from build123d import *

# Parameters (mm, degrees)
EXTRUDE_1_DEPTH     = 5
SKETCH_3_W          = 100
SKETCH_3_H          = 5
SKETCH_3_W_2        = 5
SKETCH_3_H_2        = 60
EXTRUDE_2_DEPTH     = 55
SKETCH_4_W          = 60
SKETCH_4_H          = 5
EXTRUDE_3_DEPTH     = 100
CUT_EXTRUDE_1_REACH = 89.07
FILLET_2_R          = 10
FILLET_3_R          = 10
FILLET_4_R          = 5
FILLET_5_R          = 2
CUT_EXTRUDE_2_REACH = 85.703
SKETCH_6_R          = 1.65
CUT_EXTRUDE_START   = -50
CUT_EXTRUDE_3_DEPTH = 50
EXTRUDE_4_DEPTH     = 60
SKETCH_10_W         = 7.5
SKETCH_10_H         = 18
CUT_EXTRUDE_4_DEPTH = 5


# Read off the part's stored shape, not the designer's step: 切除-拉伸3
with BuildPart() as part:
    # 草图1 → 凸台-拉伸1 (new body)
    with BuildSketch(Plane(origin=(0, 0, 0), x_dir=(1, 0, 0), z_dir=(0, 1, 0))):
        Polygon((-52.5, 35), (-52.5, -35), (52.5, -35), (52.5, -9), (-20, -9), (-20, 9), (52.5, 9), (52.5, 35), align=None)
    extrude(amount=EXTRUDE_1_DEPTH)

    # 草图3 → 凸台-拉伸2 (add)
    with BuildSketch(Plane(origin=(0, 5, 0), x_dir=(1, 0, 0), z_dir=(0, 1, 0))):
        with Locations((2.5, 32.5)):
            Rectangle(SKETCH_3_W, SKETCH_3_H)
        with Locations((-50, 32.5)):
            Rectangle(SKETCH_3_W_2, SKETCH_3_H)
        with Locations((-50, 0)):
            Rectangle(SKETCH_3_W_2, SKETCH_3_H_2)
        with Locations((2.5, -32.5)):
            Rectangle(SKETCH_3_W, SKETCH_3_H)
        with Locations((-50, -32.5)):
            Rectangle(SKETCH_3_W_2, SKETCH_3_H)
    extrude(amount=EXTRUDE_2_DEPTH)

    # 草图4 → 凸台-拉伸3 (add)
    with BuildSketch(Plane(origin=(-47.5, 0, 0), x_dir=(0, 0, -1), z_dir=(1, 0, 0))):
        with Locations((0, 57.5)):
            Rectangle(SKETCH_4_W, SKETCH_4_H)
    extrude(amount=EXTRUDE_3_DEPTH)

    # 草图5 → 切除-拉伸1 (cut, up to next)
    with BuildSketch(Plane.XZ, mode=Mode.PRIVATE) as cut_extrude_1_sk1:
        with BuildLine():
            Line((19.852941176, 10.588235294), (0, 22.5))
            ThreePointArc((0, 22.5), (-22.5, 0), (0, -22.5))
            Line((0, -22.5), (19.852941176, -10.588235294))
            ThreePointArc((19.852941176, -10.588235294), (20.252840641, -9.801655267), (20.621590627, -9))
            Line((20.621590627, -9), (-20, -9))
            Line((-20, -9), (-20, 9))
            Line((-20, 9), (20.621590627, 9))
            ThreePointArc((20.621590627, 9), (20.252840641, 9.801655267), (19.852941176, 10.588235294))
        make_face()
    cut_extrude_1_tool1 = extrude(cut_extrude_1_sk1.sketch, amount=-CUT_EXTRUDE_1_REACH, mode=Mode.PRIVATE) & part.part
    # 草图5 → 切除-拉伸1 (cut, up to next)
    with BuildSketch(Plane.XZ, mode=Mode.PRIVATE) as cut_extrude_1_sk2:
        with BuildLine():
            Line((22.5, 9), (19.852941176, 10.588235294))
            ThreePointArc((19.852941176, 10.588235294), (20.252840641, 9.801655267), (20.621590627, 9))
            Line((20.621590627, 9), (22.5, 9))
        make_face()
    cut_extrude_1_tool2 = extrude(cut_extrude_1_sk2.sketch, amount=-CUT_EXTRUDE_1_REACH, mode=Mode.PRIVATE) & part.part
    # 草图5 → 切除-拉伸1 (cut, up to next)
    with BuildSketch(Plane.XZ, mode=Mode.PRIVATE) as cut_extrude_1_sk3:
        with BuildLine():
            ThreePointArc((20.621590627, -9), (20.252840641, -9.801655267), (19.852941176, -10.588235294))
            Line((19.852941176, -10.588235294), (22.5, -9))
            Line((22.5, -9), (20.621590627, -9))
        make_face()
    cut_extrude_1_tool3 = extrude(cut_extrude_1_sk3.sketch, amount=-CUT_EXTRUDE_1_REACH, mode=Mode.PRIVATE) & part.part
    # 草图5 → 切除-拉伸1 (cut, up to next)
    with BuildSketch(Plane.XZ, mode=Mode.PRIVATE) as cut_extrude_1_sk4:
        with BuildLine():
            ThreePointArc((19.852941176, 10.588235294), (11.576154497, 19.293590829), (0, 22.5))
            Line((0, 22.5), (19.852941176, 10.588235294))
        make_face()
    cut_extrude_1_tool4 = extrude(cut_extrude_1_sk4.sketch, amount=-CUT_EXTRUDE_1_REACH, mode=Mode.PRIVATE) & part.part
    # 草图5 → 切除-拉伸1 (cut, up to next)
    with BuildSketch(Plane.XZ, mode=Mode.PRIVATE) as cut_extrude_1_sk5:
        with BuildLine():
            Line((19.852941176, -10.588235294), (0, -22.5))
            ThreePointArc((0, -22.5), (11.576154497, -19.293590829), (19.852941176, -10.588235294))
        make_face()
    cut_extrude_1_tool5 = extrude(cut_extrude_1_sk5.sketch, amount=-CUT_EXTRUDE_1_REACH, mode=Mode.PRIVATE) & part.part
    add(cut_extrude_1_tool1.solids().sort_by_distance((19.691832, 0, -9.530147))[0], mode=Mode.SUBTRACT)
    add(cut_extrude_1_tool2.solids().sort_by_distance((21.001859, 0, 9.525708))[0], mode=Mode.SUBTRACT)
    add(cut_extrude_1_tool3.solids().sort_by_distance((21.001859, 0, -9.525708))[0], mode=Mode.SUBTRACT)
    add(cut_extrude_1_tool4.solids().sort_by_distance((10.590548, 0, 17.650913))[0], mode=Mode.SUBTRACT)
    add(cut_extrude_1_tool5.solids().sort_by_distance((10.590548, 0, -17.650913))[0], mode=Mode.SUBTRACT)

    # 圆角2
    # the kernel refuses this fillet: 10 mm, written as the material it takes off along each edge
    with BuildSketch(Plane(origin=(19.852941176, -6.249770084, 10.588235294), x_dir=(-0.5108705169858321, 0, 0.8596576730737815), z_dir=(0, 1, 0))) as fillet_2_piece_1:
        with BuildLine():
            CenterArc((2.542282374, 9.989311313), FILLET_2_R, 241.685588385, 25.665066698)
            Line((-2.200814232, 1.185730531), (0, 0))
            ThreePointArc((0, 0), (1.040024608, 0.024049546), (2.080049215, 0))
        make_face()
    extrude(amount=17.499540168, mode=Mode.SUBTRACT)
    with BuildSketch(Plane(origin=(22.5, -6.924599124, 9), x_dir=(1, 0, 0), z_dir=(0, 1, 0))) as fillet_2_piece_2:
        with BuildLine():
            CenterArc((FILLET_2_R * 0.276983964948, -FILLET_2_R), FILLET_2_R, 90, 30.963756532)
            Line((-FILLET_2_R * 0.237511790479, -FILLET_2_R * 0.142507074287), (0, 0))
            Line((0, 0), (FILLET_2_R * 0.276983964948, 0))
        make_face()
    extrude(amount=18.849198247, mode=Mode.SUBTRACT)

    # 圆角3
    # the kernel refuses this fillet: 10 mm, written as the material it takes off along each edge
    with BuildSketch(Plane(origin=(22.5, -6.924599124, -9), x_dir=(1, 0, 0), z_dir=(0, 1, 0))) as fillet_3_piece_1:
        with BuildLine():
            CenterArc((FILLET_3_R * 0.276983964948, FILLET_3_R), FILLET_3_R, 239.036243468, 30.963756532)
            Line((-FILLET_3_R * 0.237511790479, FILLET_3_R * 0.142507074287), (0, 0))
            Line((0, 0), (FILLET_3_R * 0.276983964948, 0))
        make_face()
    extrude(amount=18.849198247, mode=Mode.SUBTRACT)
    with BuildSketch(Plane(origin=(19.852941176, -6.249770084, -10.588235294), x_dir=(0.857492925712544, 0, 0.5144957554275268), z_dir=(0, 1, 0))) as fillet_3_piece_2:
        with BuildLine():
            CenterArc((2.499908034, 10), FILLET_3_R, 244.334933302, 25.665066698)
            ThreePointArc((-1.83118813, 0.986587437), (-0.904187133, 0.514465931), (0, 0))
            Line((0, 0), (2.499908034, 0))
        make_face()
    extrude(amount=17.499540168, mode=Mode.SUBTRACT)

    # 圆角4
    fillet_4_edges = [part.edges().sort_by_distance(p)[0] for p in [
        (0, 0, 35),
        (0, 0, -35),
        (0, 60, -35),
        (0, 60, 35),
    ]]
    fillet(fillet_4_edges, radius=FILLET_4_R)

    # 圆角5
    fillet_5_edges = [part.edges().sort_by_distance(p)[0] for p in [
        (52.5, 5, 19.5),
        (52.5, 5, -19.5),
        (52.5, 30, -30),
        (52.5, 30, 30),
        (52.5, 55, 0),
    ]]
    fillet(fillet_5_edges, radius=FILLET_5_R)

    # 草图6 → 切除-拉伸2 (cut, up to next)
    with BuildSketch(Plane.XZ.offset(-55), mode=Mode.PRIVATE) as cut_extrude_2_sk1:
        with Locations(Location((-24.75, 24.75, 0), (0, 0, 270))):
            Circle(SKETCH_6_R)
    cut_extrude_2_tool1 = extrude(cut_extrude_2_sk1.sketch, amount=-CUT_EXTRUDE_2_REACH, mode=Mode.PRIVATE) & part.part
    # 草图6 → 切除-拉伸2 (cut, up to next)
    with BuildSketch(Plane.XZ.offset(-55), mode=Mode.PRIVATE) as cut_extrude_2_sk2:
        with Locations(Location((24.75, 24.75, 0), (0, 0, 270))):
            Circle(SKETCH_6_R)
    cut_extrude_2_tool2 = extrude(cut_extrude_2_sk2.sketch, amount=-CUT_EXTRUDE_2_REACH, mode=Mode.PRIVATE) & part.part
    # 草图6 → 切除-拉伸2 (cut, up to next)
    with BuildSketch(Plane.XZ.offset(-55), mode=Mode.PRIVATE) as cut_extrude_2_sk3:
        with Locations(Location((24.75, -24.75, 0), (0, 0, 270))):
            Circle(SKETCH_6_R)
    cut_extrude_2_tool3 = extrude(cut_extrude_2_sk3.sketch, amount=-CUT_EXTRUDE_2_REACH, mode=Mode.PRIVATE) & part.part
    # 草图6 → 切除-拉伸2 (cut, up to next)
    with BuildSketch(Plane.XZ.offset(-55), mode=Mode.PRIVATE) as cut_extrude_2_sk4:
        with Locations(Location((-24.75, -24.75, 0), (0, 0, 270))):
            Circle(SKETCH_6_R)
    cut_extrude_2_tool4 = extrude(cut_extrude_2_sk4.sketch, amount=-CUT_EXTRUDE_2_REACH, mode=Mode.PRIVATE) & part.part
    add(cut_extrude_2_tool1.solids().sort_by_distance((-24.75, 55, 24.75))[0], mode=Mode.SUBTRACT)
    add(cut_extrude_2_tool2.solids().sort_by_distance((24.75, 55, 24.75))[0], mode=Mode.SUBTRACT)
    add(cut_extrude_2_tool3.solids().sort_by_distance((24.75, 55, -24.75))[0], mode=Mode.SUBTRACT)
    add(cut_extrude_2_tool4.solids().sort_by_distance((-24.75, 55, -24.75))[0], mode=Mode.SUBTRACT)

    # 切除-拉伸3 outline → 切除-拉伸3 (cut)
    with BuildSketch(Plane.XZ.offset(CUT_EXTRUDE_START)):
        with BuildLine():
            Line((30, 19.393928679), (35.25210063, 24.75))
            Line((35.25210063, 24.75), (30.106071321, 30))
            ThreePointArc((30.106071321, 30), (17.250375047, 24.82500375), (30, 19.393928679))
        make_face()
        with BuildLine():
            Line((-14.143398282, 24.75), (-19.393398282, 30))
            Line((-19.393398282, 30), (-19.5, 30))
            Line((-19.5, 30), (-19.446699141, 30.053300859))
            ThreePointArc((-19.446699141, 30.053300859), (-32.25, 24.75), (-19.446699141, 19.446699141))
            Line((-19.446699141, 19.446699141), (-14.143398282, 24.75))
        make_face()
        with BuildLine():
            Line((-19.5, -30), (-19.393398282, -30))
            Line((-19.393398282, -30), (-14.143398282, -24.75))
            Line((-14.143398282, -24.75), (-19.446699141, -19.446699141))
            ThreePointArc((-19.446699141, -19.446699141), (-32.25, -24.75), (-19.446699141, -30.053300859))
            Line((-19.446699141, -30.053300859), (-19.5, -30))
        make_face()
        with BuildLine():
            Line((35.356601718, -24.75), (30.053300859, -19.446699141))
            ThreePointArc((30.053300859, -19.446699141), (17.25, -24.75), (30.053300859, -30.053300859))
            Line((30.053300859, -30.053300859), (30, -30))
            Line((30, -30), (30.106601718, -30))
            Line((30.106601718, -30), (35.356601718, -24.75))
        make_face()
    extrude(amount=CUT_EXTRUDE_3_DEPTH, mode=Mode.SUBTRACT)

    # 草图9 → 凸台-拉伸4 (add)
    with BuildSketch(Plane(origin=(0, 0, 30), x_dir=(-1, 0, 0), z_dir=(0, 0, -1))):
        with BuildLine():
            Line((-43, 5), (-46.75, 7.165063509))
            ThreePointArc((-46.75, 7.165063509), (-45.834936491, 6.25), (-45.5, 5))
            Line((-45.5, 5), (-43, 5))
        make_face()
        with BuildLine():
            ThreePointArc((-46.75, 7.165063509), (-49.25, 7.165063509), (-50.5, 5))
            Line((-50.5, 5), (-48, 5))
            Line((-48, 5), (-46.75, 7.165063509))
        make_face()
        with BuildLine():
            Line((-46.75, 7.165063509), (-48, 5))
            Line((-48, 5), (-45.5, 5))
            ThreePointArc((-45.5, 5), (-45.834936491, 6.25), (-46.75, 7.165063509))
        make_face()
    extrude(amount=EXTRUDE_4_DEPTH)

    # 草图10 → 切除-拉伸4 (cut)
    with BuildSketch(Plane.XZ.offset(-5)):
        with Locations((46.75, 0)):
            Rectangle(SKETCH_10_W, SKETCH_10_H)
    extrude(amount=-CUT_EXTRUDE_4_DEPTH, mode=Mode.SUBTRACT)


solid = part.part
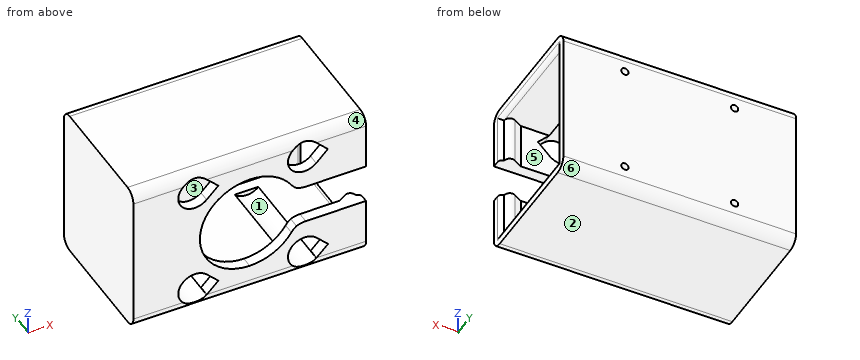
Verification items for the finished model (mm, model axes). Face numbers are marked on the shaded views. A direction names the side the tool comes from. Coordinates: 2 decimals unless noted, no trailing zeros. Order: outer loops, then holes, each group sorted by start corner. A loop starts at its lowest first (then second) coordinate and runs counter-clockwise, first axis right, second up.
1. Scan lines: line 1 (Y direction, x = -16.5, z = 20); line 2 (Z direction, x = -4, y = 50); line 3 (Z direction, x = 24, y = 58). Record each from-to range of solid material in increasing order.
Results found:
line 1: y = 0 to 5, 55 to 60
line 2: z = -35 to -30, 30 to 35
line 3: z = -34 to -26.22, -23.28 to 23.28, 26.22 to 34
2. Sectioned sample at B-B, the plane y = 30.5. Record the cut outline in (x, z).
Results found:
outline: (-52.5, -35) - (52.5, -35) - (52.5, -32) arc R2 ccw to (50.5, -30) - (30, -30) - (30.05, -30.05) arc R7.5 cw to (19.39, -30) - (-19.5, -30) - (-19.45, -30.05) arc R7.5 cw to (-30.11, -30) - (-47.5, -30) - (-47.5, 30) - (-30.11, 30) arc R7.5 cw to (-19.45, 30.05) - (-19.5, 30) - (19.39, 30) arc R7.5 cw to (30.11, 30) - (50.5, 30) arc R2 ccw to (52.5, 32) - (52.5, 35) - (-52.5, 35) - close
3. Set-up check for the marked faces 1 and 2: record each of +Z, -Z, +X, -X, +Y, -Y from which the full face is reachable in a straight line by a thin tool's end or side.
Results found:
face 1: -Y
face 2: -Z, +X, -X, +Y, -Y
4. Sectioned sample at C-C, the plane z = 0. Record the cut outline in (x, y), and give its area (3 significant figures).
Results found:
outline: (-52.5, 0) - (-22.5, 0) - (-22.5, 5) - (-47.5, 5) - (-47.5, 55) - (50.5, 55) arc R2 ccw to (52.5, 57) - (52.5, 60) - (-52.5, 60) - close
area: 924 mm2
5. Sectioned sample at D-D, the plane x = -24.75. Record the cut outline in (y, z).
Results found:
outline: (0, -17.25) - (5, -17.25) - (5, 17.25) - (0, 17.25) - close; (0.53, -32.25) arc R5 ccw to (5, -35) - (55, -35) arc R5 ccw to (60, -30) - (60, -26.4) - (55, -26.4) - (55, -30) - (50, -30) - (50, -32.25) - close; (0.53, 32.25) - (50, 32.25) - (50, 30) - (55, 30) - (55, 26.4) - (60, 26.4) - (60, 30) arc R5 ccw to (55, 35) - (5, 35) arc R5 ccw to start; (55, -23.1) - (60, -23.1) - (60, 23.1) - (55, 23.1) - close
6. Sectioned sample at A-A, the plane z = 15. Record the cut outline in (x, y), and give its area (3 significant figures).
Results found:
outline: (-52.5, 0) - (-16.77, 0) - (-16.77, 5) - (-47.5, 5) - (-47.5, 55) - (50.5, 55) arc R2 ccw to (52.5, 57) - (52.5, 60) - (-52.5, 60) - close; (16.77, 0) - (52.5, 0) - (52.5, 3) arc R2 ccw to (50.5, 5) arc R2.5 ccw to (46.75, 7.17) - (43, 5) - (16.77, 5) - close
area: 1,140 mm2
7. Release check for a two-part mould opening along Y. For the marked faces 3, 4, 5 and 6 record: +Y half, -Y half, draft (parallel to the pull), parting line (faces both ways), or undercut.
Results found:
face 3: undercut
face 4: -Y half
face 5: undercut
face 6: +Y half
8. Go/stop test with flat-tipped pins: pin 1 Ø8 at (y, z) = (34.5, -2) entering from +X; pin 2 Ø0.7 at (x, z) = (-25, 30.5) entering from -Y; pin 3 Ø3.5 at (x, y) = (36, 2.5) entering from -Z. Record where each tip stops, or that it passes through.
Results found:
pin 1: stops at x = -47.5
pin 2: stops at y = 50
pin 3: stops at z = -34.94
